Could you check a few things on this drawing? It's one solid part, dimensions in mm from its lowest x, y, z. A direction names the side the tool comes from. Coordinates: 2 decimals unless noted, no trailing zeros. Write each loop counter-clockwise with the first axis right and the second up, starting at its lowest first coordinate (ties: lowest second). Pieces come first, ordered by that corner, then holes.
Item 1: I want a section at A-A (y = 17.85). Please give me the cut outline in (x, z), and give its area (3 significant figures).
Item 2: Please list where these lines run through material, in increasing order: line 1 (X direction, y = 14.5, z = 3.75); line 2 (Y direction, x = 25.1, z = 2.1); line 3 (Y direction, x = 16.5, z = 1.15).
Item 3: I want a section at B-B (x = 11.75). Please give me the cut outline in (y, z), and give its area (3 significant figures).
Item 4: If we mould it in two halves opening along X, with no side actions, what happens to the marked faces 1, 2, 3 and 4? For each: pulls with the +X half, pulls with the -X half, needs draft (parallel to the pull), parting line crosses it, or undercut.
Item 5: For the marked faces 5 and 6, which set-ups out of +Z, -Z, +X, -X, +Y, -Y let a thin tool reach every point of the face, with its end or its side?
Item 6: I'm going to push flat-ended pins straight in: P1, Ø1.3, axis at x = 12, z = 2, coming from the -Y side; P2, Ø1.5, axis at x = 14, z = 2, coming from the -Y side; P3, Ø1.9, axis at x = 25.1, y = 28.15, coming from the +Z side. Where does each tip first touch, or does it pass through?
Item 7: I want a section at C-C (z = 1.35). Please give me the cut outline in (x, y).
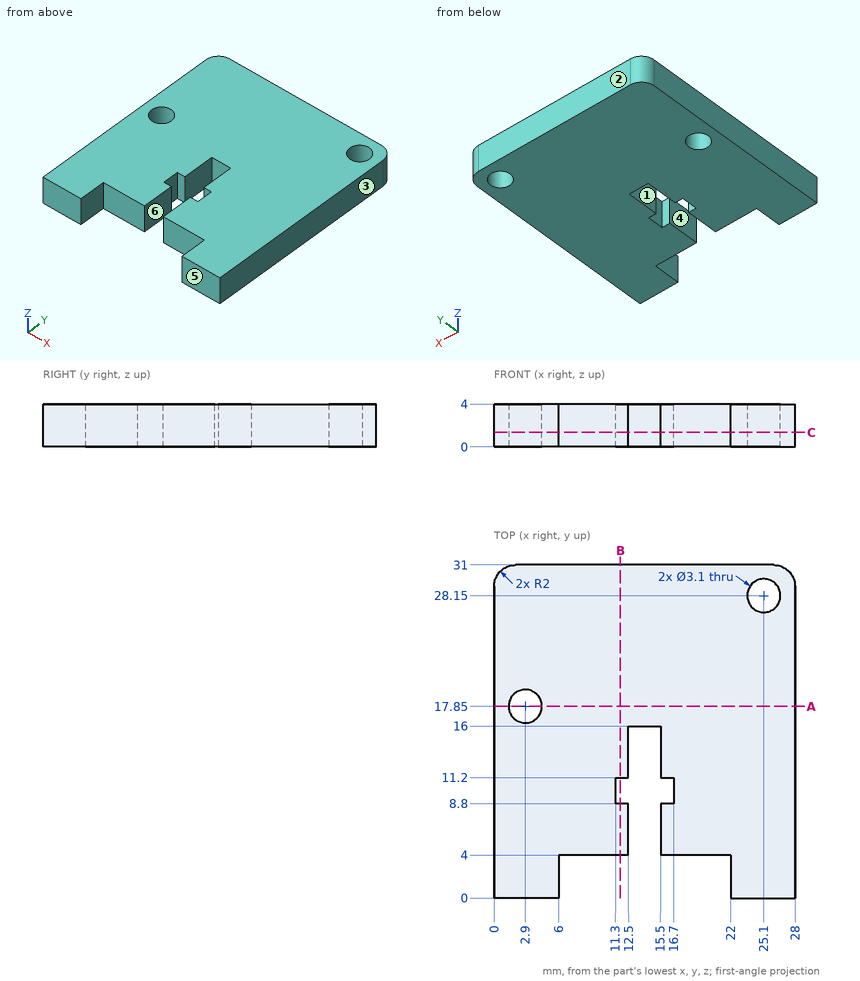
Answer:
1. outline: (0, 0) - (1.35, 0) - (1.35, 4) - (0, 4) - close; (4.45, 0) - (28, 0) - (28, 4) - (4.45, 4) - close
1. area: 99.6 mm2
2. line 1: x = 0 to 12.5, 15.5 to 28
2. line 2: y = 0 to 26.6, 29.7 to 31
2. line 3: y = 4 to 8.8, 11.2 to 31
3. outline: (4, 0) - (8.8, 0) - (8.8, 4) - (4, 4) - close; (11.2, 0) - (31, 0) - (31, 4) - (11.2, 4) - close
3. area: 98.4 mm2
4. face 1: undercut
4. face 2: needs draft
4. face 3: pulls with the +X half
4. face 4: undercut
5. face 5: +Z, -Z, +X, -X, -Y
5. face 6: +Z, -Z, -Y
6. P1: stops at y = 4
6. P2: stops at y = 16
6. P3: passes through
7. outline: (0, 0) - (6, 0) - (6, 4) - (12.5, 4) - (12.5, 8.8) - (11.3, 8.8) - (11.3, 11.2) - (12.5, 11.2) - (12.5, 16) - (15.5, 16) - (15.5, 11.2) - (16.7, 11.2) - (16.7, 8.8) - (15.5, 8.8) - (15.5, 4) - (22, 4) - (22, 0) - (28, 0) - (28, 29) arc R2 ccw to (26, 31) - (2, 31) arc R2 ccw to (0, 29) - close; hole circle Ø3.1 at (2.9, 17.85); hole circle Ø3.1 at (25.1, 28.15)
